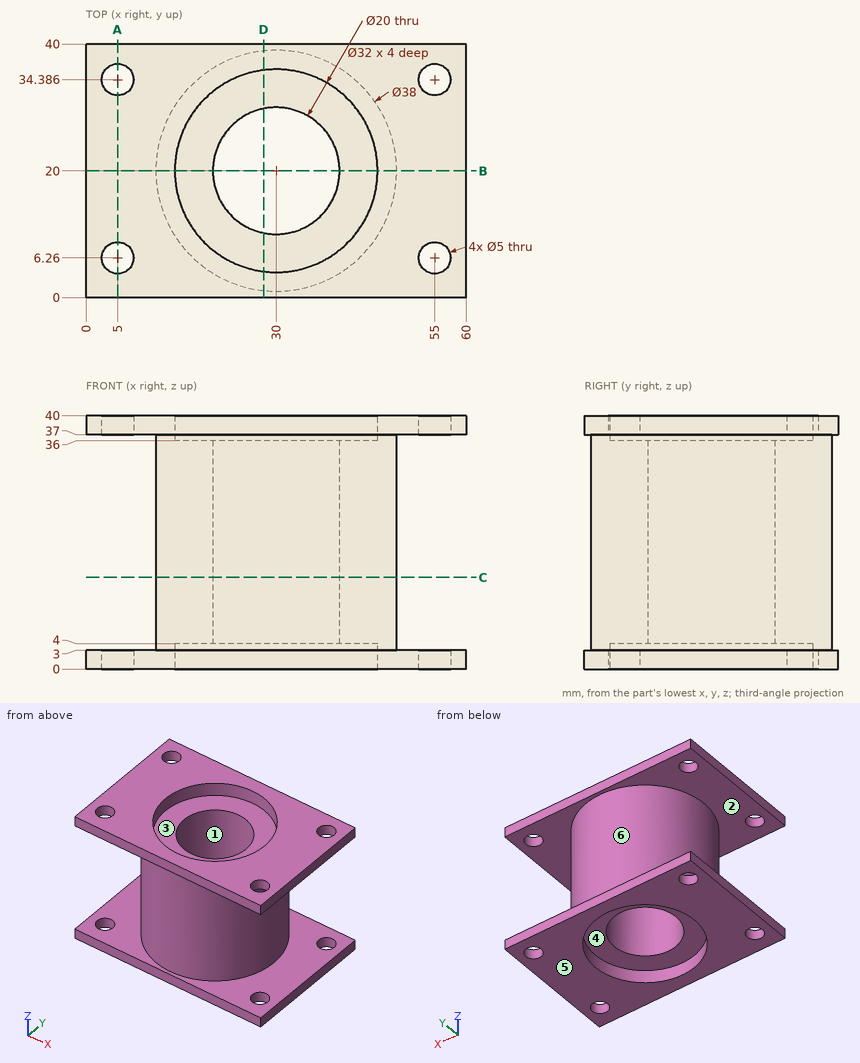
Geometry check sheet. Reference: drawing and pictorial views, mm from the part's lowest x, y, z. A direction names the side the tool comes from. Round coordinates to 2 decimals unless told otherwise and drop trailing zeros. Write each loop counter-clockwise with the first axis right and the second up, starting at its lowest first coordinate (ties: lowest second). Pieces come first, ordered by that corner, then holes.
(1) Section check D-D (x = 28). Enter the section's corners in (y, z) (1 decimal).
Returned:
outline: (0, 0) - (4.1, 0) - (4.1, 4) - (10.2, 4) - (10.2, 36) - (4.1, 36) - (4.1, 40) - (0, 40) - (0, 37) - (1.1, 37) - (1.1, 3) - (0, 3) - close; (29.8, 4) - (35.9, 4) - (35.9, 0) - (40, 0) - (40, 3) - (38.9, 3) - (38.9, 37) - (40, 37) - (40, 40) - (35.9, 40) - (35.9, 36) - (29.8, 36) - close
(2) Section check C-C (z = 14.5). Enter the section's corners in (x, y).
Returned:
outline: circle Ø38 at (30, 20); hole circle Ø20 at (30, 20)
(3) Depth check by flat-ended pin: pin 1 Ø9.5 at (x, y) = (24.5, 13) entering from -Z; pin 2 Ø5 at (x, z) = (49.5, 27) entering from -Y (1 decimal); pin 3 Ø1 at (x, z) = (13.5, 4.5) entering from -Y. Enter the tip coordinate at first touch or a pass-through.
Returned:
pin 1: stops at z = 4
pin 2: stops at y = 11.5
pin 3: stops at y = 9.75
(4) Section check A-A (x = 5). Enter the section's corners in (y, z).
Returned:
outline: (0, 0) - (3.76, 0) - (3.76, 3) - (0, 3) - close; (0, 37) - (3.76, 37) - (3.76, 40) - (0, 40) - close; (8.76, 0) - (31.89, 0) - (31.89, 3) - (8.76, 3) - close; (8.76, 37) - (31.89, 37) - (31.89, 40) - (8.76, 40) - close; (36.89, 0) - (40, 0) - (40, 3) - (36.89, 3) - close; (36.89, 37) - (40, 37) - (40, 40) - (36.89, 40) - close
(5) Mould release check, pull along Z, two halves, no side actions. Record for the marked faces 1, 2, 3 and 4: pulls with the +Z half, pulls with the -Z half, needs draft (parallel to the pull), parting line crosses it, or undercut.
Returned:
face 1: needs draft
face 2: undercut
face 3: pulls with the +Z half
face 4: pulls with the -Z half
(6) Section check B-B (y = 20). Enter the section's corners in (x, z), plus the area to 3 significant figures.
Returned:
outline: (0, 0) - (14, 0) - (14, 4) - (20, 4) - (20, 36) - (14, 36) - (14, 40) - (0, 40) - (0, 37) - (11, 37) - (11, 3) - (0, 3) - close; (40, 4) - (46, 4) - (46, 0) - (60, 0) - (60, 3) - (49, 3) - (49, 37) - (60, 37) - (60, 40) - (46, 40) - (46, 36) - (40, 36) - close
area: 756 mm2
(7) Access from +Z, -Z, +X, -X, +Y, -Y to the whole of each face (thin tool, end or side, straight path). Record for the marked faces 5 and 6.
Returned:
face 5: -Z, +X, -X, +Y, -Y
face 6: none
(8) Material ranges on line 1 (Y direction, x = 55, z = 38.85); line 2 (Z direction, x = 51.5, y = 17.5); line 3 (X direction, y = 22.5, z = 5.5) (1 decimal), recorded low to high.
Returned:
line 1: y = 0 to 3.76, 8.76 to 31.89, 36.89 to 40
line 2: z = 0 to 3, 37 to 40
line 3: x = 11.2 to 20.3, 39.7 to 48.8
